For this review, take the finished solid that the model builds, in its own axes (mm). Give positions to 0.01 mm unless a question says otherwise; leave off trailing zeros. Order: outer loops, then holes, each group sorted by start corner. A loop starts at its lowest first (then second) coordinate and runs counter-clockwise, first axis right, second up. Notation, with made-up numbers: (51.25, 46.5) - (91.25, 46.5) arc R21 cw to (91.25, 58.5) - close; hole circle Ø10 at (-8.75, -17). An arc over 180 degrees is marked (long way). Answer as a JSON object with one key per item and string values. Group by question number.
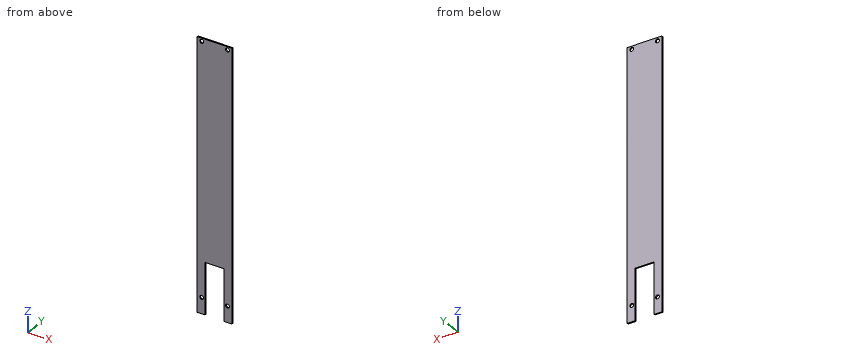
from build123d import *

# Parameters (mm, degrees)
SKETCH1_W           = 54
SKETCH1_H           = 420
BOSS_EXTRUDE1_DEPTH = 2
CUT_EXTRUDE1_REACH  = 4
SKETCH2_W           = 30
SKETCH2_H           = 80
CUT_EXTRUDE2_REACH  = 4
SKETCH3_R           = 3


with BuildPart() as part:
    # Sketch1 → Boss-Extrude1 (new body)
    with BuildSketch(Plane(origin=(0, 100, 0), x_dir=(-1, 0, 0), z_dir=(0, 1, 0))):
        with Locations((1.051745534, 184.692172039)):
            Rectangle(SKETCH1_W, SKETCH1_H)
    extrude(amount=BOSS_EXTRUDE1_DEPTH)

    # Sketch2 → Cut-Extrude1 (cut, up to next)
    with BuildSketch(Plane(origin=(0, 102, 0), x_dir=(-1, 0, 0), z_dir=(0, 1, 0)), mode=Mode.PRIVATE) as cut_extrude1_sk1:
        with Locations((1.051745534, 14.692172039)):
            Rectangle(SKETCH2_W, SKETCH2_H)
    cut_extrude1_tool1 = extrude(cut_extrude1_sk1.sketch, amount=-CUT_EXTRUDE1_REACH, mode=Mode.PRIVATE) & part.part
    add(cut_extrude1_tool1.solids().sort_by_distance((-1.051746, 102, 14.692172))[0], mode=Mode.SUBTRACT)

    # Sketch3 → Cut-Extrude2 (cut, up to next)
    with BuildSketch(Plane(origin=(0, 102, 0), x_dir=(-1, 0, 0), z_dir=(0, 1, 0)), mode=Mode.PRIVATE) as cut_extrude2_sk1:
        with Locations((-18.948254466, -0.307827961)):
            Circle(SKETCH3_R)
    cut_extrude2_tool1 = extrude(cut_extrude2_sk1.sketch, amount=-CUT_EXTRUDE2_REACH, mode=Mode.PRIVATE) & part.part
    add(cut_extrude2_tool1.solids().sort_by_distance((18.948254, 102, -0.307828))[0], mode=Mode.SUBTRACT)
    # Sketch3 → Cut-Extrude2 (cut, up to next)
    with BuildSketch(Plane(origin=(0, 102, 0), x_dir=(-1, 0, 0), z_dir=(0, 1, 0)), mode=Mode.PRIVATE) as cut_extrude2_sk2:
        with Locations((21.051745534, -0.307827961)):
            Circle(SKETCH3_R)
    cut_extrude2_tool2 = extrude(cut_extrude2_sk2.sketch, amount=-CUT_EXTRUDE2_REACH, mode=Mode.PRIVATE) & part.part
    add(cut_extrude2_tool2.solids().sort_by_distance((-21.051746, 102, -0.307828))[0], mode=Mode.SUBTRACT)
    # Sketch3 → Cut-Extrude2 (cut, up to next)
    with BuildSketch(Plane(origin=(0, 102, 0), x_dir=(-1, 0, 0), z_dir=(0, 1, 0)), mode=Mode.PRIVATE) as cut_extrude2_sk3:
        with Locations((21.051745534, 389.692172039)):
            Circle(SKETCH3_R)
    cut_extrude2_tool3 = extrude(cut_extrude2_sk3.sketch, amount=-CUT_EXTRUDE2_REACH, mode=Mode.PRIVATE) & part.part
    add(cut_extrude2_tool3.solids().sort_by_distance((-21.051746, 102, 389.692172))[0], mode=Mode.SUBTRACT)
    # Sketch3 → Cut-Extrude2 (cut, up to next)
    with BuildSketch(Plane(origin=(0, 102, 0), x_dir=(-1, 0, 0), z_dir=(0, 1, 0)), mode=Mode.PRIVATE) as cut_extrude2_sk4:
        with Locations((-18.948254466, 389.692172039)):
            Circle(SKETCH3_R)
    cut_extrude2_tool4 = extrude(cut_extrude2_sk4.sketch, amount=-CUT_EXTRUDE2_REACH, mode=Mode.PRIVATE) & part.part
    add(cut_extrude2_tool4.solids().sort_by_distance((18.948254, 102, 389.692172))[0], mode=Mode.SUBTRACT)


solid = part.part
1) For pin 1 (1 mm diameter, centred on x = -5.5, y = 101, fed in from -Z), flat-tipped, find the tip position at first contact; note if it passes through.
2) Consider section C-C (x = 5.5). Give the boundary of the cut face in (y, z).
3) Consider section A-A (z = 7). Give the boundary of the cut face in (x, y), plus the area to 3 significant figures.
4) Consider section B-B (y = 101.45). Give the boundary of the cut face in (x, z), plus the area to 3 significant figures.
5) For line 1 (X direction, y = 101.25, z = 18.5); line 2 (Z direction, x = 20, y = 101.95); line 3 (Z direction, x = -7.5, y = 100.2), list the stretches that pass through material, from the lowest coordinate up.
Result set:
{
 "1": {"pin 1": "stops at z = 54.69"},
 "2": {"outline": "(100, 54.69) - (102, 54.69) - (102, 394.69) - (100, 394.69) - close"},
 "3": {"outline": "(-28.05, 100) - (-16.05, 100) - (-16.05, 102) - (-28.05, 102) - close; (13.95, 100) - (25.95, 100) - (25.95, 102) - (13.95, 102) - close", "area": "48.0 mm2"},
 "4": {"outline": "(-28.05, -25.31) - (-16.05, -25.31) - (-16.05, 54.69) - (13.95, 54.69) - (13.95, -25.31) - (25.95, -25.31) - (25.95, 394.69) - (-28.05, 394.69) - close; hole circle Ø6 at (-21.05, -0.31); hole circle Ø6 at (-21.05, 389.69); hole circle Ø6 at (18.95, -0.31); hole circle Ø6 at (18.95, 389.69)", "area": "20,200 mm2"},
 "5": {"line 1": "x = -28.05 to -16.05, 13.95 to 25.95", "line 2": "z = -25.31 to -3.12, 2.5 to 386.88, 392.5 to 394.69", "line 3": "z = 54.69 to 394.69"}
}
